from build123d import *

# Parameters (mm, degrees)
SKETCH1_R      = 4
SKETCH1_R_2    = 2.05
EXTRUDE1_DEPTH = 5
CHAMFER2_SIZE  = 0.25


with BuildPart() as part:
    # Sketch1 → Extrude1 (new body)
    with BuildSketch(Plane.XY):
        Circle(SKETCH1_R)
        Circle(SKETCH1_R_2, mode=Mode.SUBTRACT)
    extrude(amount=EXTRUDE1_DEPTH)

    # Chamfer2
    chamfer2_edges = [part.edges().sort_by_distance(p)[0] for p in [
        (-4, 0, 0),
        (-4, 0, 5),
        (-2.05, 0, 0),
        (-2.05, 0, 5),
    ]]
    chamfer(chamfer2_edges, length=CHAMFER2_SIZE)


solid = part.part
Input: part model. Units: mm. Frame: model coordinates. Round coordinates to 2 decimals unless told otherwise and drop trailing zeros. Order: outer loops, then holes, each group sorted by start corner. A loop starts at its lowest first (then second) coordinate and runs counter-clockwise, first axis right, second up. Notation, with made-up numbers: (23, 43) - (49, 43) arc R23 ccw to (49, 54) - close; hole circle Ø4 at (29, 8). An arc over 180 degrees is marked (long way). Use a Markdown table: item, result.
1. Material intervals for probe 1 along Y at (x, z) = (0, 2.5); probe 2 along X at (y, z) = (0.5, 1.8); probe 3 along X at (y, z) = (1.75, 4.3), sorted ascending.
Evaluation:
| item | result |
|---|---|
| probe 1 | -4 to -2.05, 2.05 to 4 |
| probe 2 | -3.97 to -1.99, 1.99 to 3.97 |
| probe 3 | -3.6 to -1.07, 1.07 to 3.6 |
2. Mould query, pull axis X, two halves, no side actions, for faces 1 (the face through (-2, -2, 0)), 2 (the face through (-0.867, -3.905, 2.468)), 3 (the face through (-0.267, 2.033, 2.468)). Classes: +X half, -X half, draft (parallel to the pull), parting line (faces both ways), or undercut.
Evaluation:
| item | result |
|---|---|
| face 1 | draft |
| face 2 | parting line |
| face 3 | undercut |
3. Section A-A on x = 0. Return the cut outline in (y, z), then the cut area to 4 significant figures.
Evaluation:
| item | result |
|---|---|
| outline | (-4, 0.25) - (-3.75, 0) - (-2.3, 0) - (-2.05, 0.25) - (-2.05, 4.75) - (-2.3, 5) - (-3.75, 5) - (-4, 4.75) - close; (2.05, 0.25) - (2.3, 0) - (3.75, 0) - (4, 0.25) - (4, 4.75) - (3.75, 5) - (2.3, 5) - (2.05, 4.75) - close |
| area | 19.25 mm^2 |
4. First-contact query: pin 1 (2 mm diameter, centred on x = 2.5, z = 4, fed in from +Y); pin 2 (2 mm diameter, centred on y = -2, z = 4, fed in from -X); pin 3 (3 mm diameter, centred on x = 2.5, z = 4, fed in from -Y). Flat tips, straight axial feed; report the tip coordinate or a pass-through.
Evaluation:
| item | result |
|---|---|
| pin 1 | y = 3.71 |
| pin 2 | x = -3.87 |
| pin 3 | y = -3.87 |
5. Section B-B on z = 1.65. Return the cut outline in (x, y), then the cut area to 3 significant figures.
Evaluation:
| item | result |
|---|---|
| outline | circle Ø8 at (0, 0); hole circle Ø4.1 at (0, 0) |
| area | 37.1 mm^2 |
